from build123d import *

# Parameters (mm, degrees)
F1_DEPTH = 15
F2_R     = 3
F3_DEPTH = 50
F4_SIZE  = 0.5
F7_D     = 2.4
F7_DEPTH = 20
F7_TIP   = 0.7210327428


with BuildPart() as f1:
    # F0 (on Front) → F1 (new body)
    with BuildSketch(Plane.XZ):
        with BuildLine():
            Line((-2, 2.2360679775), (-2, -2.2360679775))
            ThreePointArc((-2, -2.2360679775), (0, -3), (2, -2.2360679775))
            Line((2, -2.2360679775), (2, 2.2360679775))
            ThreePointArc((2, 2.2360679775), (0, 3), (-2, 2.2360679775))
        make_face()
    extrude(amount=-F1_DEPTH)

    # F2 (on Front) → F3 (join)
    with BuildSketch(Plane.XZ):
        Circle(F2_R)
    extrude(amount=F3_DEPTH)

    # F4
    f4_edges = [f1.edges().sort_by_distance(p)[0] for p in [
        (-3, -50, 0),
        (0, 15, 3),
        (-2, 15, 0),
        (0, 15, -3),
        (2, 15, 0),
    ]]
    chamfer(f4_edges, length=F4_SIZE)

    # F7
    with Locations(Plane(origin=(0, 15, 0), x_dir=(-1, 0, 0), z_dir=(0, 1, 0))):
        with Locations((0, 0)):
            Hole(F7_D / 2, depth=F7_DEPTH)
            with Locations((0, 0, -(F7_DEPTH + F7_TIP / 2))):  # 118° drill point
                Cone(0, F7_D / 2, F7_TIP, mode=Mode.SUBTRACT)


solid = f1.part
CAD build for the part. Positions are in the model's coordinates, mm. A direction names the side the tool comes from. Round coordinates to 2 decimals unless told otherwise and drop trailing zeros. Loops run counter-clockwise (first coordinate to the right, second up) from the corner with the lowest first, then second, coordinate; pieces in that order, holes last.
(1) Wall check: line 1 along Z through (x, y) = (0, 4.5); line 2 along X through (y, z) = (6.5, 0). Give the ranges that are in metal, low to high.
(2) Cut at A-A (y = 9.5). Give the cut face in (x, z).
(3) Drop flat-ended pins along their axis: pin 1 (1.1 mm diameter, centred on x = -2.5, z = -1, fed in from +Y); pin 2 (3.5 mm diameter, centred on y = 10, z = 0, fed in from +X); pin 3 (1 mm diameter, centred on x = -1, y = -10.5, fed in from -Z). Give the stop position or say it passes through.
(4) Two-plate mould, pull along Z, no slides. Class faces 1 (the conical face through (-0.03, 14.86, -2.64)), 2 (the cylindrical face through (0.65, 4.86, 1.01)), 3 (the flat face through (2.4, 0, 0)): +Z half, -Z half, draft (parallel to the pull), parting line (faces both ways), or undercut.
(5) Which spindle directions (+Z, -Z, +X, -X, +Y, -Y) get a long thin tool onto all of the face, cutting with end or side? Do faces 4 (the conical face through (0.03, 14.86, 2.64)), 5 (the flat face through (2, 7, 0)), 6 (the flat face through (-2, 7, 0)). Say none if no direction does.
(6) Cut at B-B (y = -42.5). Give the cut face in (x, z), plus the area to 3 significant figures.
Findings below:
1. line 1: z = -3 to -1.2, 1.2 to 3
1. line 2: x = -2 to -1.2, 1.2 to 2
2. outline: (-2, -2.24) arc R3 ccw to (2, -2.24) - (2, 2.24) arc R3 ccw to (-2, 2.24) - close; hole circle Ø2.4 at (0, 0)
3. pin 1: stops at y = 14.55
3. pin 2: stops at x = 2
3. pin 3: stops at z = -2.96
4. face 1: -Z half
4. face 2: undercut
4. face 3: draft
5. face 4: +Z, +Y
5. face 5: +Z, -Z, +X, +Y
5. face 6: +Z, -Z, -X, +Y
6. outline: circle Ø6 at (0, 0)
6. area: 28.3 mm2
